Input: part model. Units: mm. Frame: model coordinates. A direction names the side the tool comes from. Round coordinates to 2 decimals unless told otherwise and drop trailing zeros. Order: outer loops, then holes, each group sorted by start corner. A loop starts at its lowest first (then second) coordinate and runs counter-clockwise, first axis right, second up. Notation, with made-up numbers: (46.5, 46.25) -> (95.5, 46.25) arc R31 cw to (95.5, 75.25) -> close; hole circle Ø11 at (-9, 27.25). An arc over 180 degrees is marked (long way). Answer as CSV lines item,"result". Start each with the question number.
1) Access query for faces 1 (the face through (0, 1.27, 4)), 2 (the face through (0, 0, 0)). Directions: +Z, -Z, +X, -X, +Y, -Y. A direction counts if a zero-diameter tool reaches every point of the face in a straight line with its end or side. Return the directions, or none.
2) Section query B-B, the plane z = -4. Output: boundary loops of the cut face in (x, y).
3) First-contact query: P1, Ø1, axis at y = 2, z = 3.5, coming from the -X side; P2, Ø1.5, axis at y = 3, z = 2, coming from the +X side; P3, Ø2, axis at x = -3, z = -1, coming from the +Y side. Flat tips, straight axial feed; report the tip coordinate or a pass-through.
4) Line query: L1, parallel to Y at x = -3, z = 3; L2, parallel to Z at x = 0, y = 2.75; L3, parallel to X at y = 2.5, z = -2.5. Output: solid intervals per line, ascending.
5) Section query A-A, the plane y = 2.1. Output: boundary loops of the cut face in (x, z), and give its area (3 significant figures).
Autodesk Inventor part; units mm, degrees
ref_plane "YZ Plane" through (0, 0, 0) normal (1, 0, 0) x (0, 1, 0)
ref_plane "XZ Plane" through (0, 0, 0) normal (0, 1, 0) x (-1, 0, 0)
ref_plane "XY Plane" through (0, 0, 0) normal (0, 0, 1) x (1, 0, 0)
sketch "Sketch1" plane through (0, 0, 0) normal (0, 1, 0) x (-1, 0, 0)
  circle A0 centre (0, 0) radius 3.683
  circle A1 centre (0, 0) radius 4.953
  dimension "d0" = 7.366
  dimension "d1" = 9.906
extrude "Extrusion1" add sketch "Sketch1" along normal blind 5.715 contours A0
extrude "Extrusion2" add sketch "Sketch1" along normal blind 1.27
fillet "Fillet1" radius 1.905 1 edges at (3.683, 5.715, 0)
properties part number "Button_switch"
Findings:
1,face 1,"+Y"
1,face 2,"+Z, -Z, +X, -X, -Y"
2,outline,"(-2.92, 0) -> (2.92, 0) -> (2.92, 1.27) -> (-2.92, 1.27) -> close"
3,P1,"stops at x = -2.14"
3,P2,"stops at x = 3.46"
3,P3,"stops at y = 5.68"
4,L1,"y = 0 to 1.27"
4,L2,"z = -3.68 to 3.68"
4,L3,"x = -2.7 to 2.7"
5,outline,"circle Ø7.37 at (0, 0)"
5,area,"42.6 mm^2"
